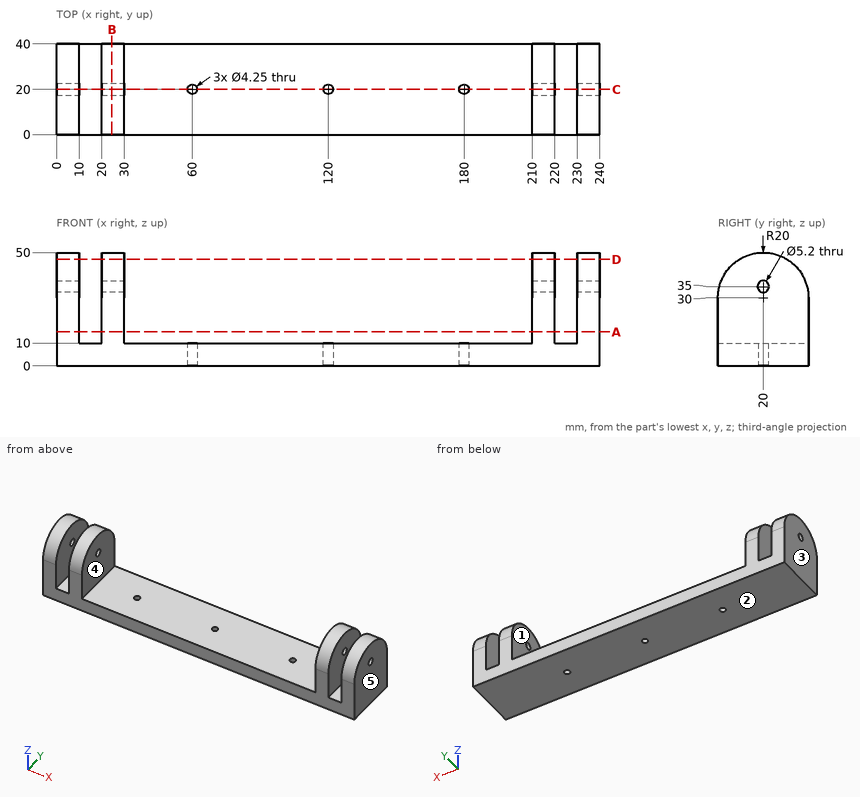
Here's the drawing with two shaded views (mm, measured from the low corner). I have some questions. A direction names the side the tool comes from. Coordinates: 2 decimals unless noted, no trailing zeros. Write each loop counter-clockwise with the first axis right and the second up, starting at its lowest first coordinate (ties: lowest second). Pieces come first, ordered by that corner, then holes. Notation, with made-up numbers: M -28.75,-25 L -5.75,-25 A10 ccw -5.75,-18 Z; hole C 81,65.25 d5. An arc over 180 degrees is marked long. Write item = value, one per line. Start each with the question number.
Q1. On a 3-axis mill with a long thin cutter (end or side, diameter ignored), from which of +Z, -Z, +X, -X, +Y, -Y can I reach the whole of each face in a straight line? I mean the marked faces 4 and 5. Say none if no direction works.
Q2. I'm going to push flat-ended pins straight in: pin 1 (5 mm diameter, centred on x = 110.5, y = 14, fed in from +Z); pin 2 (2 mm diameter, centred on x = 113.5, y = 8, fed in from -Z); pin 3 (11 mm diameter, centred on x = 225, y = 16, fed in from +Z). Where does each tip first touch, or does it pass through?
Q3. If we section it at A-A, the plane z = 15: Write out the boundary of the cut face in (x, y), then the cut area to 3 significant figures.
Q4. If we section it at D-D, the plane z = 47: Write out the boundary of the cut face in (x, y).
Q5. If we section it at B-B, the plane x = 24.5: Write out the boundary of the cut face in (y, z), then the cut area to 3 significant figures.
Q6. If we section it at C-C, the plane y = 20: State how many separate pieces and enclosed holes the cut face has, then the cut area to 3 significant figures.
Q7. Thinking about a two-plate mould opening in X: for the marked faces 1, 2 and 3, which applies, released by +X, released by -X, zero draft, split by the parting line, or undercut?
Q8. If I drill on L1, parallel to X at y = 38.5, z = 35.5; L2, parallel to Y at x = 120, z = 2 (3 decimals); L3, parallel to Z at x = 88, y = 10, over which ranges is the centre line in solid material (lowest first)? Write a range as [from, to].
Check sheet entries:
q1.face_4 = +Z, +Y, -Y
q1.face_5 = +Z, -Z, +X, +Y, -Y
q2.pin_1 = 10
q2.pin_2 = 0
q2.pin_3 = 49.93
q3.outline = M 0,0 L 10,0 L 10,40 L 0,40 Z; M 20,0 L 30,0 L 30,40 L 20,40 Z; M 210,0 L 220,0 L 220,40 L 210,40 Z; M 230,0 L 240,0 L 240,40 L 230,40 Z
q3.area = 1,600 mm²
q4.outline = M 0,9.46 L 10,9.46 L 10,30.54 L 0,30.54 Z; M 20,9.46 L 30,9.46 L 30,30.54 L 20,30.54 Z; M 210,9.46 L 220,9.46 L 220,30.54 L 210,30.54 Z; M 230,9.46 L 240,9.46 L 240,30.54 L 230,30.54 Z
q5.outline = M 0,0 L 40,0 L 40,30 A20 ccw 0,30 Z; hole C 20,35 d5.2
q5.area = 1,810 mm²
q6.separate_pieces = 8
q6.enclosed_holes = 0
q6.area = 3,660 mm²
q7.face_1 = undercut
q7.face_2 = zero draft
q7.face_3 = released by -X
q8.L1 = [0, 10], [20, 30], [210, 220], [230, 240]
q8.L2 = [0, 17.875], [22.125, 40]
q8.L3 = [0, 10]
